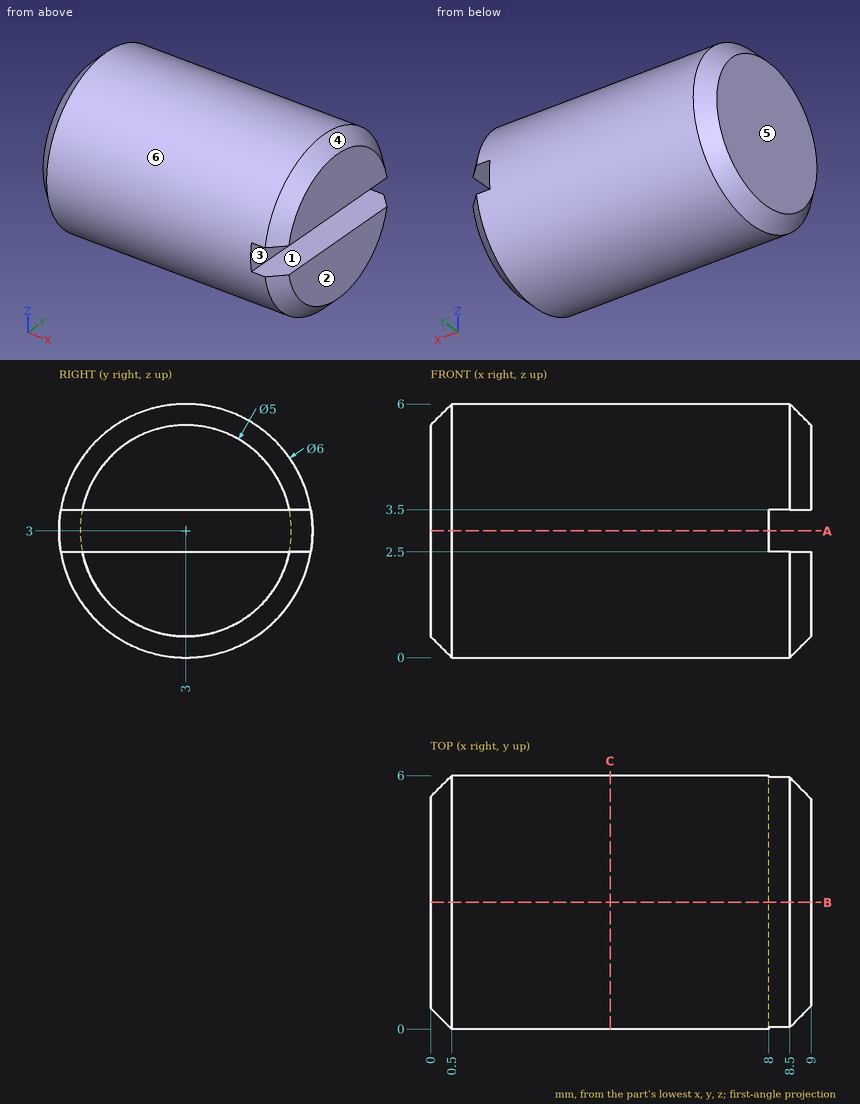
Verification items for this drawing (mm, ordinates from the low corner). A direction names the side the tool comes from. Round coordinates to 2 decimals unless told otherwise and drop trailing zeros. Order: outer loops, then holes, each group sorted by start corner. A loop starts at its lowest first (then second) coordinate and runs counter-clockwise, first axis right, second up. Notation, with made-up numbers: M -23.75,69.25 L 34.25,69.25 A13 cw 34.25,81.25 Z; hole C 49.5,76.25 d5. An arc over 180 degrees is marked long. Answer in a Markdown table with one row per item. Add a question column.
Item 1: Material ranges on L1, parallel to X at y = 4.85, z = 2.95; L2, parallel to Y at x = 7, z = 2.5; L3, parallel to Y at x = 6.25, z = 0.6, recorded low to high. Write a range as [from, to].
Item 2: Sectioned sample at A-A, the plane z = 3. Enter the section's corners in (x, y), plus the area to 4 significant figures.
Item 3: Sectioned sample at B-B, the plane y = 3. Enter the section's corners in (x, z).
Item 4: Draft check along Z on the marked faces 3, 4, 5 and 6. Enter one of: released by +Z, released by -Z, zero draft, split by the parting line, or undercut.
Item 5: Sectioned sample at C-C, the plane x = 4.25. Enter the section's corners in (y, z).
Item 6: Depth check by flat-ended pin: pin 1 Ø0.5 at (x, y) = (8.5, 1.5) entering from +Z; pin 2 Ø1.5 at (x, z) = (7, 5) entering from -Y; pin 3 Ø0.8 at (x, y) = (8.5, 3.5) entering from -Z; pin 4 Ø0.5 at (y, z) = (4, 3) entering from +X. Enter the tip coordinate at first touch or a pass-through.
Item 7: Set-up check for the marked faces 1 and 2: record each of +Z, -Z, +X, -X, +Y, -Y from which the full face is reachable in a straight line by a thin tool's end or side.
Filled in:
| question | item | result |
|---|---|---|
| 1 | L1 | x = [0, 8] |
| 1 | L2 | y = [0.04, 5.96] |
| 1 | L3 | y = [1.2, 4.8] |
| 2 | outline | M 0,0.5 L 0.5,0 L 8,0 L 8,6 L 0.5,6 L 0,5.5 Z |
| 2 | area | 47.75 mm² |
| 3 | outline | M 0,0.5 L 0.5,0 L 8.5,0 L 9,0.5 L 9,2.5 L 8,2.5 L 8,3.5 L 9,3.5 L 9,5.5 L 8.5,6 L 0.5,6 L 0,5.5 Z |
| 4 | face 3 | undercut |
| 4 | face 4 | released by +Z |
| 4 | face 5 | zero draft |
| 4 | face 6 | split by the parting line |
| 5 | outline | C 3,3 d6 |
| 6 | pin 1 | stops at z = 5.73 |
| 6 | pin 2 | stops at y = 0.27 |
| 6 | pin 3 | stops at z = 0 |
| 6 | pin 4 | stops at x = 8 |
| 7 | face 1 | +X, +Y, -Y |
| 7 | face 2 | +Z, -Z, +X, +Y, -Y |
